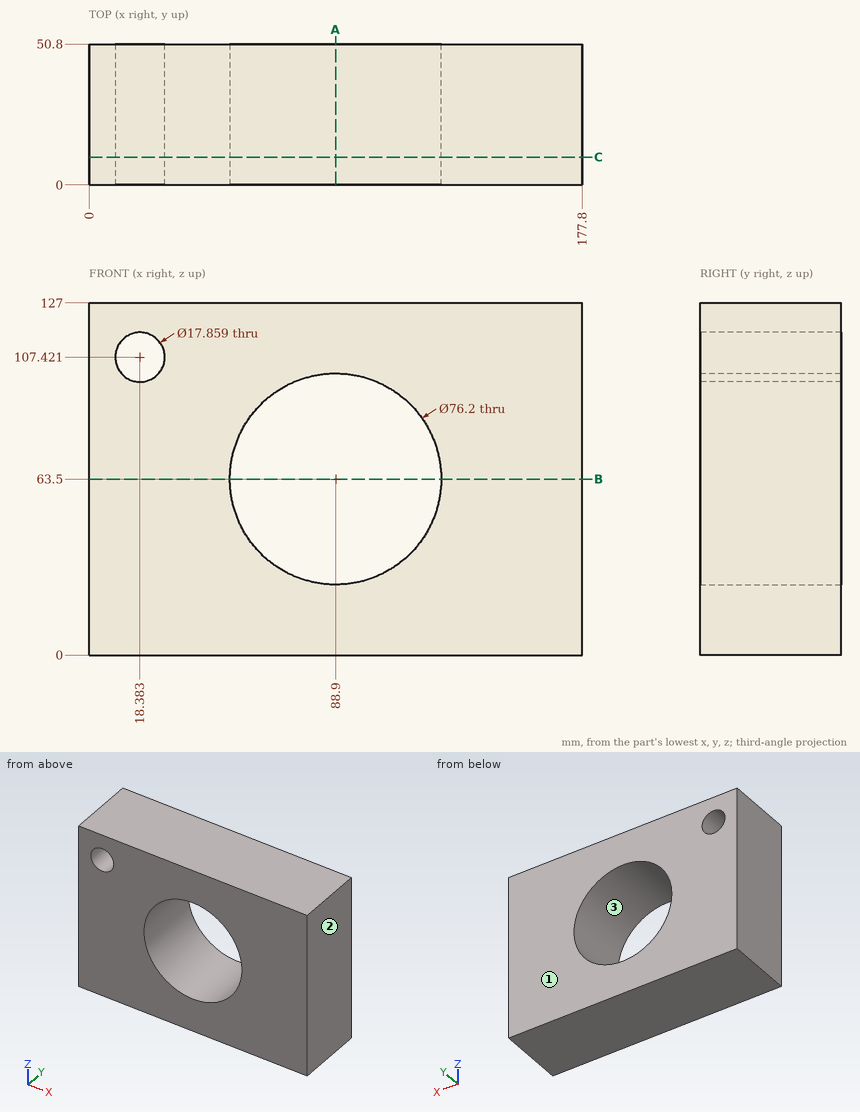
The figure shows three views and two pictorial views of one solid part (mm, origin at its lowest corner). Answer the questions. Give positions to 0.01 mm unless a question says otherwise; leave off trailing zeros. Write each loop counter-clockwise with the first axis right and the second up, starting at its lowest first coordinate (ties: lowest second). Pieces come first, ordered by that corner, then holes. Notation, with made-up numbers: (-25, -26.75) -> (25, -26.75) arc R30 ccw to (25, 1.25) -> close; hole circle Ø10 at (66, 31). An arc over 180 degrees is marked (long way). Answer as a JSON object with one key per item and string values.
1) For a pull along X with two mould halves and no side action, classify the marked faces 1, 2 and 3 as pulls with the +X half, pulls with the -X half, needs draft (parallel to the pull), parting line crosses it, or undercut.
Findings below:
{"face 1": "needs draft", "face 2": "pulls with the +X half", "face 3": "undercut"}
2) Section A-A on x = 88.9 is taken. Write down the section's boundary in (y, z).
Findings below:
{"outline": "(0, 0) -> (50.8, 0) -> (50.8, 25.4) -> (0, 25.4) -> close; (0, 101.6) -> (50.8, 101.6) -> (50.8, 127) -> (0, 127) -> close"}
3) Section C-C on y = 10 is taken. Write down the section's boundary in (x, z).
Findings below:
{"outline": "(0, 0) -> (177.8, 0) -> (177.8, 127) -> (0, 127) -> close; hole circle Ø17.86 at (18.38, 107.42); hole circle Ø76.2 at (88.9, 63.5)"}
4) Straight lines are drawn through the part: probe 1 along Z at (x, y) = (88.9, 16); probe 2 along X at (y, z) = (19.5, 62.5); probe 3 along X at (y, z) = (43.5, 114) (1 decimal). For each, find the intervals that lie inside material, in ascending order. Write a range as from..to.
Findings below:
{"probe 1": "z = 0..25.4, 101.6..127", "probe 2": "x = 0..50.81, 126.99..177.8", "probe 3": "x = 0..12.3, 24.4..177.8"}
5) Section B-B on z = 63.5 is taken. Write down the section's boundary in (x, y), then the cut area to 3 significant figures.
Findings below:
{"outline": "(0, 0) -> (50.8, 0) -> (50.8, 50.8) -> (0, 50.8) -> close; (127, 0) -> (177.8, 0) -> (177.8, 50.8) -> (127, 50.8) -> close", "area": "5,160 mm^2"}
